Design review of the part built by this model. Coordinates are the model's own, in mm. A direction names the side the tool comes from. Coordinates: 2 decimals unless noted, no trailing zeros. Order: outer loops, then holes, each group sorted by start corner. A loop starts at its lowest first (then second) coordinate and runs counter-clockwise, first axis right, second up.
from build123d import *

# Parameters (mm, degrees)
SKETCH_1_R          = 3.25
SKETCH_1_R_2        = 2.25
SKETCH_1_R_3        = 1.75
EXTRUDE_1_DEPTH     = 0.3
SKETCH_1_4_R        = 2.25
SKETCH_1_4_R_2      = 1.75
EXTRUDE_2_DEPTH     = 5
CUT_EXTRUDE_1_DEPTH = 3.2
FILLET_1_R          = 0.05


with BuildPart() as part:
    # Sketch 1 → Extrude 1 (new body)
    with BuildSketch(Plane.XY):
        Circle(SKETCH_1_R)
        Circle(SKETCH_1_R_2, mode=Mode.SUBTRACT)
        Circle(SKETCH_1_R_2)
        Circle(SKETCH_1_R_3, mode=Mode.SUBTRACT)
    extrude(amount=EXTRUDE_1_DEPTH)

    # Sketch 1_4 → Extrude 2 (add)
    with BuildSketch(Plane.XY):
        Circle(SKETCH_1_4_R)
        Circle(SKETCH_1_4_R_2, mode=Mode.SUBTRACT)
    extrude(amount=-EXTRUDE_2_DEPTH)

    # Sketch 2 → Cut-Extrude 1 (cut)
    with BuildSketch(Plane(origin=(0, 0, -5), x_dir=(-1, 0, 0), z_dir=(0, 0, -1))):
        with BuildLine():
            ThreePointArc((-0.65, 2.154065923), (-2.25, 0), (-0.65, -2.154065923))
            Line((-0.65, -2.154065923), (-0.65, -1.624807681))
            ThreePointArc((-0.65, -1.624807681), (-1.75, 0), (-0.65, 1.624807681))
            Line((-0.65, 1.624807681), (-0.65, 2.154065923))
        make_face()
        with BuildLine():
            Line((0.65, -1.624807681), (0.65, -2.154065923))
            ThreePointArc((0.65, -2.154065923), (1.806239187, -1.341640786), (2.25, 0))
            ThreePointArc((2.25, 0), (1.806239187, 1.341640786), (0.65, 2.154065923))
            Line((0.65, 2.154065923), (0.65, 1.624807681))
            ThreePointArc((0.65, 1.624807681), (1.449137675, 0.981070844), (1.75, 0))
            ThreePointArc((1.75, 0), (1.449137675, -0.981070844), (0.65, -1.624807681))
        make_face()
    extrude(amount=-CUT_EXTRUDE_1_DEPTH, mode=Mode.SUBTRACT)

    # Fillet 1
    fillet_1_edges = [part.edges().sort_by_distance(p)[0] for p in [
        (1.806239187, 1.341640786, -1.8),
        (0.65, -1.889436802, -5),
        (0.65, 1.889436802, -5),
        (0, -2.25, -5),
        (0, -1.75, -5),
        (-0.65, -1.889436802, -5),
        (-0.65, 1.889436802, -5),
        (-2.25, 0, -1.8),
        (-3.25, 0, 0),
        (-3.25, 0, 0.3),
        (0, 2.25, -5),
        (0, 1.75, -5),
    ]]
    fillet(fillet_1_edges, radius=FILLET_1_R)


solid = part.part
1. Add section C-C (z = -0.85). Give the boundary of the cut face in (x, y).
2. Add section B-B (x = 0). Give the boundary of the cut face in (y, z).
3. To check wall thickness, follow line 1 (Y direction, x = 0, z = 0.25); line 2 (Y direction, x = 0, z = -2.85); line 3 (Z direction, x = -2.25, y = 1.75). State the ranges of each line that lie inside material, in increasing order.
4. Insertion check: pin 1 (0.8 mm diameter, centred on x = 1.5, y = 0.5, fed in from -Z); pin 2 (1.5 mm diameter, centred on y = 1.5, z = -1.5, fed in from -X); pin 3 (1 mm diameter, centred on x = -0.5, z = -1, fed in from -Y). Each pin has a flat end and moves straight along its axis. Give the tip position at first contact, or say it passes through.
5. For faces 1 (the flat face through (1.4, -2.1, 0)), 2 (the flat face through (1.4, -1.4, 0.3)), 3 (the flat face through (2, 0, -1.8)), 4 (the flat face through (-2, 0, -1.8)), list the 3-axis set-ups (+Z, -Z, +X, -X, +Y, -Y) from which the entire face can be reached by the end or side of a thin tool; tool diameter is ignored.
6. Add section A-A (z = -1.95). Give the boundary of the cut face in (x, y), and give its area (3 significant figures).
Solution:
1. outline: circle Ø4.5 at (0, 0); hole circle Ø3.5 at (0, 0)
2. outline: (-3.25, 0.05) arc R0.05 ccw to (-3.2, 0) - (-2.25, 0) - (-2.25, -4.95) arc R0.05 ccw to (-2.2, -5) - (-1.8, -5) arc R0.05 ccw to (-1.75, -4.95) - (-1.75, 0.3) - (-3.2, 0.3) arc R0.05 ccw to (-3.25, 0.25) - close; (1.75, -4.95) arc R0.05 ccw to (1.8, -5) - (2.2, -5) arc R0.05 ccw to (2.25, -4.95) - (2.25, 0) - (3.2, 0) arc R0.05 ccw to (3.25, 0.05) - (3.25, 0.25) arc R0.05 ccw to (3.2, 0.3) - (1.75, 0.3) - close
3. line 1: y = -3.25 to -1.75, 1.75 to 3.25
3. line 2: y = -2.25 to -1.75, 1.75 to 2.25
3. line 3: z = 0 to 0.3
4. pin 1: stops at z = -1.8
4. pin 2: stops at x = -2.12
4. pin 3: stops at y = -2.25
5. face 1: -Z
5. face 2: +Z, +X, -X, +Y, -Y
5. face 3: -Z, +X, +Y, -Y
5. face 4: -Z, -X, +Y, -Y
6. outline: (-0.65, -2.15) arc R2.25 ccw to (0.65, -2.15) - (0.65, -1.62) arc R1.75 cw to (-0.65, -1.62) - close; (-0.65, 1.62) arc R1.75 cw to (0.65, 1.62) - (0.65, 2.15) arc R2.25 ccw to (-0.65, 2.15) - close
6. area: 1.32 mm2
